from build123d import *

# Parameters (mm, degrees)
F7_R      = 6.35
F8_DEPTH  = 254
F10_W     = 25.4
F10_H     = 6.35
F9_W      = 50.8
F9_H      = 6.35
F11_D     = 3.175
F11_DEPTH = 6.3510001
F5_D      = 3.175
F6_R      = 0.79375


with BuildPart() as f8:
    # F7 (on line) → F8 (new body)
    with BuildSketch(Plane(origin=(-127, 0, 0), x_dir=(0, -1, 0), z_dir=(-1, 0, 0))):
        with Locations((0, -6.35)):
            Circle(F7_R)
    extrude(amount=-F8_DEPTH)

    # F10 (on line) → F4 section 0
    with BuildSketch(Plane.XY.offset(-12.7)):
        Rectangle(F10_W, F10_H)
    # F9 (on line) → F4 section 1
    with BuildSketch(Plane.XY):
        Rectangle(F9_W, F9_H)
    loft(mode=Mode.SUBTRACT)

    # F11 (through all, one way)
    with BuildSketch(Plane.XZ):
        with Locations((-9.525, -6.35), (9.525, -6.35)):
            Circle(F11_D / 2)
    extrude(amount=-F11_DEPTH, mode=Mode.SUBTRACT)

    # F5 (through all)
    with Locations(Plane(origin=(0, 0, 0), x_dir=(1, 0, 0), z_dir=(0, 1, 0))):
        with Locations((-9.525, 6.35), (9.525, 6.35)):
            Hole(F5_D / 2)

    # F6
    f6_edges = [f8.edges().sort_by_distance(p)[0] for p in [
        (127, 6.35, -6.35),
        (-127, 6.35, -6.35),
    ]]
    fillet(f6_edges, radius=F6_R)


solid = f8.part
Verification items for the finished model (mm, model axes). A direction names the side the tool comes from. Coordinates: 2 decimals unless noted, no trailing zeros. Order: outer loops, then holes, each group sorted by start corner. A loop starts at its lowest first (then second) coordinate and runs counter-clockwise, first axis right, second up. Notation, with made-up numbers: M -4,6 L 3,6 A16 cw 3,27 Z; hole C 82,-1 d4. An arc over 180 degrees is marked long. One line per item, written item: value. Start each with the question number.
Item 1: Mould release check, pull along X, two halves, no side actions. Record for faces 1 (the flat face through (19.1, 0, -6.3)), 2 (the flat face through (-127, 0, -6)), 3 (the flat face through (127, 0, -6)): released by +X, released by -X, zero draft, split by the parting line, or undercut.
Item 2: Sectioned sample at A-A (y = 0). Enter the section's corners in (x, z).
Item 3: Access from +Z, -Z, +X, -X, +Y, -Y to the whole of each face (thin tool, end or side, straight path). Record for faces 4 (the cylindrical face through (-1.767, -3.414, -0.996)), 5 (the flat face through (-19.1, 0, -6.3)).
Item 4: Gauge pin test, flat end, axial feed: pin 1 (1 mm diameter, centred on x = 94.5, y = -4.5, fed in from -Z). Record the tip position at first contact, or that the pin passes through.
Item 5: Scan lines: probe 1 along X at (y, z) = (-5, -6.35); probe 2 along X at (y, z) = (-3.5, -7.75); probe 3 along X at (y, z) = (0, -10). Record each from-to range of solid material in increasing order.
Item 6: Sectioned sample at B-B (x = 99). Enter the section's corners in (y, z), then the cut area to 3 significant figures.
Conclusion:
1. face 1: undercut
1. face 2: released by -X
1. face 3: released by +X
2. outline: M -127,-11.91 A0.79 ccw -126.21,-12.7 L -12.7,-12.7 L -25.4,0 L -126.21,0 A0.79 ccw -127,-0.79 Z; M 12.7,-12.7 L 126.21,-12.7 A0.79 ccw 127,-11.91 L 127,-0.79 A0.79 ccw 126.21,0 L 25.4,0 Z
3. face 4: +X, -X
3. face 5: +Z
4. pin 1: stops at z = -11.28
5. probe 1: x = -127 to -11.11, -7.94 to 7.94, 11.11 to 127
5. probe 2: x = -127 to -10.27, -8.78 to 8.78, 10.27 to 127
5. probe 3: x = -127 to -15.4, 15.4 to 127
6. outline: C 0,-6.35 d12.7
6. area: 127 mm^2
